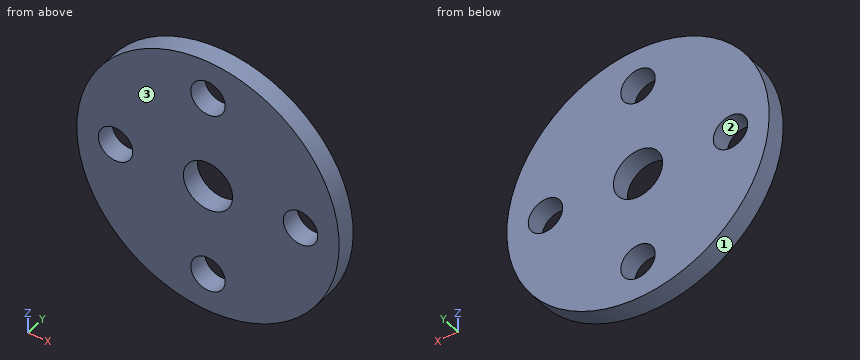
```python
from build123d import *

# Parameters (mm, degrees)
SKETCH_1_R          = 16
EXTRUDE_1_DEPTH     = 2.4
CUT_EXTRUDE_2_REACH = 24.754
SKETCH_4_R          = 2.1
CUT_EXTRUDE_3_REACH = 24.754
SKETCH_2_R          = 3


with BuildPart() as part:
    # 草圖1 → 填料-伸長1 (new body)
    with BuildSketch(Plane(origin=(0, 0, 0), x_dir=(1, 0, 0), z_dir=(0, 1, 0))):
        with Locations(Location((0, 0, 0), (0, 0, 270))):
            Circle(SKETCH_1_R)
    extrude(amount=EXTRUDE_1_DEPTH)

    # 草圖4 → 除料-伸長2 (cut, up to next)
    with BuildSketch(Plane(origin=(0, 2.4, 0), x_dir=(1, 0, 0), z_dir=(0, 1, 0)), mode=Mode.PRIVATE) as cut_extrude_2_sk1:
        with Locations(Location((0, 11.29, 0), (0, 0, 270))):
            Circle(SKETCH_4_R)
    cut_extrude_2_tool1 = extrude(cut_extrude_2_sk1.sketch, amount=-CUT_EXTRUDE_2_REACH, mode=Mode.PRIVATE) & part.part
    # 草圖4 → 除料-伸長2 (cut, up to next)
    with BuildSketch(Plane(origin=(0, 2.4, 0), x_dir=(1, 0, 0), z_dir=(0, 1, 0)), mode=Mode.PRIVATE) as cut_extrude_2_sk2:
        with Locations(Location((11.29, 0, 0), (0, 0, 270))):
            Circle(SKETCH_4_R)
    cut_extrude_2_tool2 = extrude(cut_extrude_2_sk2.sketch, amount=-CUT_EXTRUDE_2_REACH, mode=Mode.PRIVATE) & part.part
    # 草圖4 → 除料-伸長2 (cut, up to next)
    with BuildSketch(Plane(origin=(0, 2.4, 0), x_dir=(1, 0, 0), z_dir=(0, 1, 0)), mode=Mode.PRIVATE) as cut_extrude_2_sk3:
        with Locations(Location((0, -11.29, 0), (0, 0, 270))):
            Circle(SKETCH_4_R)
    cut_extrude_2_tool3 = extrude(cut_extrude_2_sk3.sketch, amount=-CUT_EXTRUDE_2_REACH, mode=Mode.PRIVATE) & part.part
    # 草圖4 → 除料-伸長2 (cut, up to next)
    with BuildSketch(Plane(origin=(0, 2.4, 0), x_dir=(1, 0, 0), z_dir=(0, 1, 0)), mode=Mode.PRIVATE) as cut_extrude_2_sk4:
        with Locations(Location((-11.29, 0, 0), (0, 0, 270))):
            Circle(SKETCH_4_R)
    cut_extrude_2_tool4 = extrude(cut_extrude_2_sk4.sketch, amount=-CUT_EXTRUDE_2_REACH, mode=Mode.PRIVATE) & part.part
    add(cut_extrude_2_tool1.solids().sort_by_distance((0, 2.4, -11.29))[0], mode=Mode.SUBTRACT)
    add(cut_extrude_2_tool2.solids().sort_by_distance((11.29, 2.4, 0))[0], mode=Mode.SUBTRACT)
    add(cut_extrude_2_tool3.solids().sort_by_distance((0, 2.4, 11.29))[0], mode=Mode.SUBTRACT)
    add(cut_extrude_2_tool4.solids().sort_by_distance((-11.29, 2.4, 0))[0], mode=Mode.SUBTRACT)

    # 草圖2 → 除料-伸長3 (cut, up to next)
    with BuildSketch(Plane(origin=(0, 2.4, 0), x_dir=(1, 0, 0), z_dir=(0, 1, 0)), mode=Mode.PRIVATE) as cut_extrude_3_sk1:
        with Locations(Location((0, 0, 0), (0, 0, 270))):
            Circle(SKETCH_2_R)
    cut_extrude_3_tool1 = extrude(cut_extrude_3_sk1.sketch, amount=-CUT_EXTRUDE_3_REACH, mode=Mode.PRIVATE) & part.part
    add(cut_extrude_3_tool1.solids().sort_by_distance((0, 2.4, 0))[0], mode=Mode.SUBTRACT)


solid = part.part
```
Build history of the part. All positions in model axes, mm. Face numbers are marked on the shaded views. Coordinates: 2 decimals unless noted, no trailing zeros. Order: outer loops, then holes, each group sorted by start corner. A loop starts at its lowest first (then second) coordinate and runs counter-clockwise, first axis right, second up. Notation, with made-up numbers: (-14.5, 71.25) -> (44.5, 71.25) arc R20 ccw to (44.5, 78.25) -> close; hole circle Ø11 at (12.25, 27.25). An arc over 180 degrees is marked (long way). Answer in a Markdown table with one row per item. Add a question column.
Q1. Band-saw the part on A-A, the plane z = 0. List the corners of the cut face in (x, y).
Q2. Band-saw the part on D-D, the plane y = 0.75. List the corners of the cut face in (x, z), then the cut area to 3 significant figures.
Q3. Mould opens along Z. For the marked faces 1, 2 and 3 say: +Z half, -Z half, draft (parallel to the pull), parting line (faces both ways), or undercut.
Q4. Band-saw the part on C-C, the plane z = 11.29. List the corners of the cut face in (x, y).
Q5. Band-saw the part on B-B, the plane x = 0. List the corners of the cut face in (y, z).
Q6. Wall check: line 1 along X through (y, z) = (1.1, 0); line 2 along Z through (x, y) = (-1.5, 1.05); line 3 along X through (y, z) = (1.9, -0.5). Give the ranges that are in metal, low to high. Write a range as [from, to].
Q7. Drop flat-ended pins along their axis: pin 1 (5 mm diameter, centred on x = 11.29, z = 0, fed in from +Y); pin 2 (3.5 mm diameter, centred on x = 0, z = 0, fed in from +Y). Give the stop position or say it passes through.
Answers follow:
| question | item | result |
|---|---|---|
| 1 | outline | (-16, 0) -> (-13.39, 0) -> (-13.39, 2.4) -> (-16, 2.4) -> close; (-9.19, 0) -> (-3, 0) -> (-3, 2.4) -> (-9.19, 2.4) -> close; (3, 0) -> (9.19, 0) -> (9.19, 2.4) -> (3, 2.4) -> close; (13.39, 0) -> (16, 0) -> (16, 2.4) -> (13.39, 2.4) -> close |
| 2 | outline | circle Ø32 at (0, 0); hole circle Ø4.2 at (-11.29, 0); hole circle Ø6 at (0, 0); hole circle Ø4.2 at (0, -11.29); hole circle Ø4.2 at (0, 11.29); hole circle Ø4.2 at (11.29, 0) |
| 2 | area | 721 mm^2 |
| 3 | face 1 | parting line |
| 3 | face 2 | undercut |
| 3 | face 3 | draft |
| 4 | outline | (-11.34, 0) -> (-2.1, 0) -> (-2.1, 2.4) -> (-11.34, 2.4) -> close; (2.1, 0) -> (11.34, 0) -> (11.34, 2.4) -> (2.1, 2.4) -> close |
| 5 | outline | (0, -16) -> (2.4, -16) -> (2.4, -13.39) -> (0, -13.39) -> close; (0, -9.19) -> (2.4, -9.19) -> (2.4, -3) -> (0, -3) -> close; (0, 3) -> (2.4, 3) -> (2.4, 9.19) -> (0, 9.19) -> close; (0, 13.39) -> (2.4, 13.39) -> (2.4, 16) -> (0, 16) -> close |
| 6 | line 1 | [-16, -13.39], [-9.19, -3], [3, 9.19], [13.39, 16] |
| 6 | line 2 | [-15.93, -12.76], [-9.82, -2.6], [2.6, 9.82], [12.76, 15.93] |
| 6 | line 3 | [-15.99, -13.33], [-9.25, -2.96], [2.96, 9.25], [13.33, 15.99] |
| 7 | pin 1 | y = 2.4 |
| 7 | pin 2 | through |
